Can you work these out from the drawing? Everything is in mm from the part's minimum corner. Round coordinates to 2 decimals unless told otherwise and drop trailing zeros. Write each loop counter-clockwise with the first axis right and the second up, starting at its lowest first coordinate (ties: lowest second). Pieces come first, ordered by that corner, then holes.
Q1. If we section it at B-B (x = 21.5): Please give me the cut outline in (y, z), plus the area to 3 significant figures.
Q2. Please list where these lines run through material, in increasing order: line 1 along Y through (x, z) = (18, 0.75); line 2 along Z through (x, y) = (7, 6); line 3 along Z through (x, y) = (17, 4).
Q3. I'm going to push flat-ended pins straight in: pin 1 Ø1 at (x, z) = (11, 1.5) entering from -Y; pin 2 Ø1.3 at (x, z) = (16, 1) entering from +Y. Where does each tip first touch, or does it pass through?
Q4. If we section it at A-A (y = 4.75): Give the number of separate pieces and of enclosed holes in the cut face, plus the area to 3 significant figures.
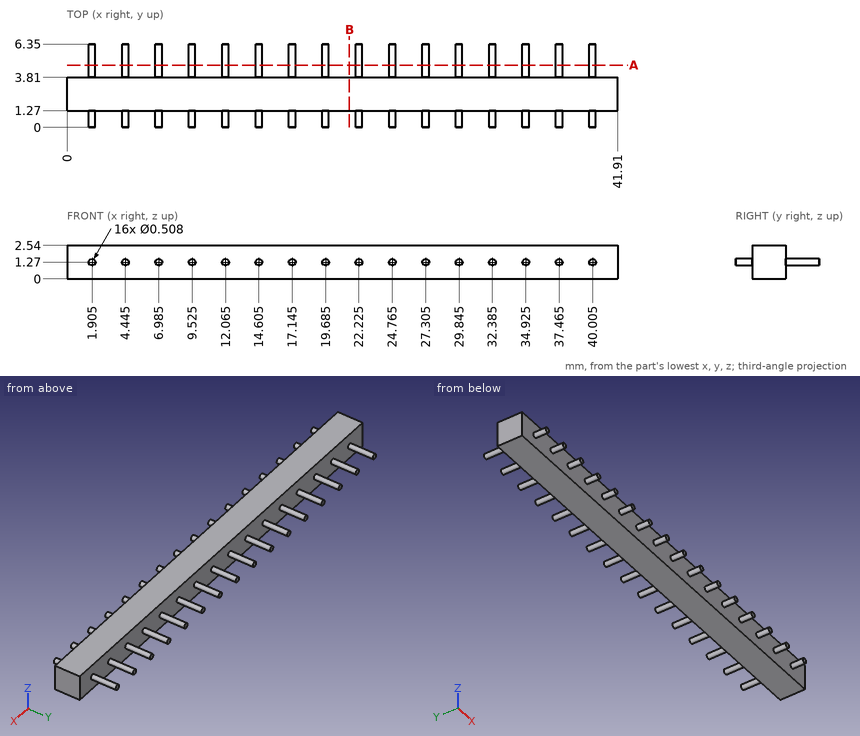
A:
1. outline: (1.27, 0) - (3.81, 0) - (3.81, 2.54) - (1.27, 2.54) - close
1. area: 6.45 mm2
2. line 1: y = 1.27 to 3.81
2. line 2: z = 1.02 to 1.52
2. line 3: z = 1.06 to 1.48
3. pin 1: stops at y = 1.27
3. pin 2: stops at y = 3.81
4. separate pieces: 16
4. enclosed holes: 0
4. area: 3.24 mm2
